Work out the finished part from the listing and answer in its coordinate system (mm). A direction names the side the tool comes from. Give positions to 0.01 mm unless a question says otherwise; leave off trailing zeros. Write each loop counter-clockwise with the first axis right and the second up, starting at its lowest first coordinate (ties: lowest second). Pieces come first, ordered by that corner, then holes. Notation, with made-up numbers: (13, 70) -> (19, 70) arc R29 cw to (19, 96) -> close; hole circle Ø3 at (-0.75, 40.5). An arc over 180 degrees is marked (long way). Use a Markdown table: item, result. Add a question column.
Q1. Each of these flat-tipped pins is pushed along its axis until it touches: pin 1 Ø3 at (x, z) = (-21.5, 25) entering from +Y; pin 2 Ø13.5 at (x, z) = (57, 21.5) entering from +Y; pin 3 Ø1.5 at (x, z) = (35.5, 26.5) entering from +Y. Where does it stop, or does it pass through?
Q2. Section B-B, the plane y = 32 is taken. Give the vertices of the cut face in (x, z).
Q3. Section D-D, the plane x = -3.5 is taken. Give the vertices of the cut face in (y, z), plus the area to 3 significant figures.
Q4. Section C-C, the plane z = 13 is taken. Give the vertices of the cut face in (x, y) (1 decimal).
Q5. Section A-A, the plane x = 42 is taken. Give the vertices of the cut face in (y, z).
Q6. For faces 1 (the face through (49, 13, 25)), 2 (the face through (5.42, 39.63, 29.71)), 3 (the face through (-49.074, 6.591, 40.999)), determine the directions among +Z, -Z, +X, -X, +Y, -Y from which every point of the face is accessible in a straight line to the end or side of a thin tool.
Q7. For a pull along Z with two mould halves and no side action, classify faces 4 (the face through (-36, 14, 38)), 5 (the face through (49.581, 6.591, 24.794)), 6 (the face through (41, 0, 19)) as pulls with the +Z half, pulls with the -Z half, needs draft (parallel to the pull), parting line crosses it, or undercut.
Q8. Consider line 1 (Z direction, x = -52, y = 34); line 2 (Z direction, x = 52, y = 6); line 3 (X direction, y = 14.5, z = 33). Determine where each line is inside the solid, lowest interval first.
from build123d import *

# Parameters (mm, degrees)
SKETCH1_R           = 4.5
BOSS_EXTRUDE1_DEPTH = 9
BOSS_EXTRUDE2_DEPTH = 51
SKETCH2_R           = 4.5
CUT_EXTRUDE1_DEPTH  = 51
BOSS_EXTRUDE4_START = -51
BOSS_EXTRUDE4_DEPTH = 51
CUT_EXTRUDE2_START  = -13
CUT_EXTRUDE2_DEPTH  = 13


with BuildPart() as part:
    # Sketch1 → Boss-Extrude1 (new body)
    with BuildSketch(Plane.XY):
        with BuildLine():
            Line((-63.686733312, 13), (-37.828560639, 13))
            ThreePointArc((-37.828560639, 13), (-35.993988141, 17.448003259), (-33.638618871, 21.643551476))
            ThreePointArc((-33.638618871, 21.643551476), (4.802775087, 39.710620135), (37.828560639, 13))
            Line((37.828560639, 13), (63.686733312, 13))
            ThreePointArc((63.686733312, 13), (48.281028578, 43.519447141), (19.519221296, 62))
            Line((19.519221296, 62), (-19.519221296, 62))
            ThreePointArc((-19.519221296, 62), (-48.281028578, 43.519447141), (-63.686733312, 13))
        make_face()
        with Locations((-41, 32)):
            Circle(SKETCH1_R, mode=Mode.SUBTRACT)
        with Locations((41, 32)):
            Circle(SKETCH1_R, mode=Mode.SUBTRACT)
    extrude(amount=BOSS_EXTRUDE1_DEPTH)

    # Sketch1_3 → Boss-Extrude2 (add)
    with BuildSketch(Plane.XY):
        with BuildLine():
            Line((-65, 13), (-65, 0))
            Line((-65, 0), (-26.9625, 0))
            ThreePointArc((-26.9625, 0), (0, 26.9625), (26.9625, 0))
            Line((26.9625, 0), (65, 0))
            Line((65, 0), (65, 13))
            Line((65, 13), (37.828560639, 13))
            ThreePointArc((37.828560639, 13), (0, 40), (-37.828560639, 13))
            Line((-37.828560639, 13), (-65, 13))
        make_face()
    extrude(amount=BOSS_EXTRUDE2_DEPTH)

    # Sketch2 → Cut-Extrude1 (cut)
    with BuildSketch(Plane(origin=(0, 13, 0), x_dir=(1, 0, 0), z_dir=(0, 1, 0))):
        with BuildLine():
            Line((-37.828560639, -51), (-60.639049437, -30.714258841))
            ThreePointArc((-60.639049437, -30.714258841), (-63.859756378, -26.324112946), (-65, -21))
            Line((-65, -21), (-65, -51))
            Line((-65, -51), (-37.828560639, -51))
        make_face()
        with Locations(Location((-52, -21, 0), (0, 0, 180))):
            Circle(SKETCH2_R)
        with BuildLine():
            Line((60.639049437, -30.714258841), (37.828560639, -51))
            Line((37.828560639, -51), (65, -51))
            Line((65, -51), (65, -21))
            ThreePointArc((65, -21), (63.859756378, -26.324112946), (60.639049437, -30.714258841))
        make_face()
        with Locations(Location((52, -21, 0), (0, 0, 180))):
            Circle(SKETCH2_R)
    extrude(amount=-CUT_EXTRUDE1_DEPTH, mode=Mode.SUBTRACT)

    # Sketch3 → Boss-Extrude4 (add)
    with BuildSketch(Plane.XY.offset(51).offset(BOSS_EXTRUDE4_START)):
        with BuildLine():
            ThreePointArc((-36.211228808, 16.992554492), (-33.954723298, 16.194730784), (-33, 14))
            ThreePointArc((-33, 14), (-34.674421243, 11.308747325), (-37.828560639, 11.621688416))
            Line((-37.828560639, 11.621688416), (-37.828560639, 6.211780307))
            ThreePointArc((-37.828560639, 6.211780307), (-31.031523629, 7.729892939), (-28, 14))
            ThreePointArc((-28, 14), (-29.562180142, 18.749155239), (-33.638618871, 21.643551476))
            ThreePointArc((-33.638618871, 21.643551476), (-35.002260619, 19.360830343), (-36.211228808, 16.992554492))
        make_face()
        with BuildLine():
            ThreePointArc((-37.828560639, 11.621688416), (-38.87258348, 14.86502263), (-36.211228808, 16.992554492))
            ThreePointArc((-36.211228808, 16.992554492), (-35.002260619, 19.360830343), (-33.638618871, 21.643551476))
            ThreePointArc((-33.638618871, 21.643551476), (-43.720483455, 16.09621927), (-37.828560639, 6.211780307))
            Line((-37.828560639, 6.211780307), (-37.828560639, 11.621688416))
        make_face()
        with BuildLine():
            ThreePointArc((-37.828560639, 11.621688416), (-34.674421243, 11.308747325), (-33, 14))
            ThreePointArc((-33, 14), (-33.954723298, 16.194730784), (-36.211228808, 16.992554492))
            ThreePointArc((-36.211228808, 16.992554492), (-37.073679723, 15.018064849), (-37.828560639, 13))
            Line((-37.828560639, 13), (-37.828560639, 11.621688416))
        make_face()
        with BuildLine():
            ThreePointArc((-37.828560639, 13), (-37.073679723, 15.018064849), (-36.211228808, 16.992554492))
            ThreePointArc((-36.211228808, 16.992554492), (-38.87258348, 14.86502263), (-37.828560639, 11.621688416))
            Line((-37.828560639, 11.621688416), (-37.828560639, 13))
        make_face()
    extrude(amount=BOSS_EXTRUDE4_DEPTH)

    # Sketch3_3 → Cut-Extrude2 (cut)
    with BuildSketch(Plane.XY.offset(51).offset(CUT_EXTRUDE2_START)):
        with BuildLine():
            ThreePointArc((-37.828560639, 11.621688416), (-34.674421243, 11.308747325), (-33, 14))
            ThreePointArc((-33, 14), (-33.954723298, 16.194730784), (-36.211228808, 16.992554492))
            ThreePointArc((-36.211228808, 16.992554492), (-37.073679723, 15.018064849), (-37.828560639, 13))
            Line((-37.828560639, 13), (-37.828560639, 11.621688416))
        make_face()
        with BuildLine():
            ThreePointArc((-37.828560639, 13), (-37.073679723, 15.018064849), (-36.211228808, 16.992554492))
            ThreePointArc((-36.211228808, 16.992554492), (-38.87258348, 14.86502263), (-37.828560639, 11.621688416))
            Line((-37.828560639, 11.621688416), (-37.828560639, 13))
        make_face()
    extrude(amount=CUT_EXTRUDE2_DEPTH, mode=Mode.SUBTRACT)


solid = part.part
Result set:
| question | item | result |
|---|---|---|
| 1 | pin 1 | stops at y = 34.64 |
| 1 | pin 2 | stops at y = 13 |
| 1 | pin 3 | stops at y = 19.81 |
| 2 | outline | (-56.58, 0) -> (-45.5, 0) -> (-45.5, 9) -> (-56.58, 9) -> close; (-36.5, 0) -> (36.5, 0) -> (36.5, 9) -> (24, 9) -> (24, 51) -> (-24, 51) -> (-24, 9) -> (-36.5, 9) -> close; (45.5, 0) -> (56.58, 0) -> (56.58, 9) -> (45.5, 9) -> close |
| 3 | outline | (26.73, 0) -> (62, 0) -> (62, 9) -> (39.85, 9) -> (39.85, 51) -> (26.73, 51) -> close |
| 3 | area | 868 mm2 |
| 4 | outline | (-65, 0) -> (-27, 0) arc R27 cw to (27, 0) -> (65, 0) -> (65, 13) -> (37.8, 13) arc R40 ccw to (-33.6, 21.6) arc R8 ccw to (-43.9, 13) -> (-65, 13) -> close |
| 5 | outline | (0, 0) -> (27.61, 0) -> (27.61, 9) -> (13, 9) -> (13, 47.29) -> (0, 47.29) -> close; (36.39, 0) -> (49.61, 0) -> (49.61, 9) -> (36.39, 9) -> close |
| 6 | face 1 | +Z, +X, +Y |
| 6 | face 2 | +Z, +Y |
| 6 | face 3 | +Z, -X, -Y |
| 7 | face 4 | pulls with the +Z half |
| 7 | face 5 | undercut |
| 7 | face 6 | needs draft |
| 8 | line 1 | z = 0 to 9 |
| 8 | line 2 | z = 0 to 16.5, 25.5 to 38.4 |
| 8 | line 3 | x = -43.98 to -22.73, 22.73 to 37.28 |
